from build123d import *

# Parameters (mm, degrees)
F0_R     = 3
F1_DEPTH = 0.8
F3_DEPTH = 2


with BuildPart() as f1:
    # F0 (on Top) → F1 (new body)
    with BuildSketch(Plane.XY):
        with BuildLine():
            Line((-2, 10.345446), (0, 10.345446))
            Line((0, 10.345446), (2, 10.345446))
            Line((2, 10.345446), (5.554248, 10.345446))
            Line((5.554248, 10.345446), (16, 10.345446))
            Line((16, 10.345446), (26.5, -2.654554))
            Line((26.5, -2.654554), (28.31125, -0.122547))
            Line((28.31125, -0.122547), (18.033634, 12.60212))
            ThreePointArc((18.033634, 12.60212), (17.339915, 13.150071), (16.477752, 13.345446))
            Line((16.477752, 13.345446), (0, 13.345446))
            Line((0, 13.345446), (-16.477752, 13.345446))
            ThreePointArc((-16.477752, 13.345446), (-17.339915, 13.150071), (-18.033634, 12.60212))
            Line((-18.033634, 12.60212), (-28.31125, -0.122547))
            Line((-28.31125, -0.122547), (-26.5, -2.654554))
            Line((-26.5, -2.654554), (-16, 10.345446))
            Line((-16, 10.345446), (-5.554248, 10.345446))
            Line((-5.554248, 10.345446), (-2, 10.345446))
        make_face()
        with Locations((0, 1.345446)):
            Circle(F0_R)
    extrude(amount=F1_DEPTH)

    # F2 (on face) → F3 (join)
    with BuildSketch(Plane(origin=(0, 0, 0), x_dir=(1, 0, 0), z_dir=(0, 0, -1))):
        with BuildLine():
            Line((-26.5, 2.654554), (-28.31125, 0.122547))
            Line((-28.31125, 0.122547), (-18.033634, -12.60212))
            ThreePointArc((-18.033634, -12.60212), (-17.339915, -13.150071), (-16.477752, -13.345446))
            Line((-16.477752, -13.345446), (16.477752, -13.345446))
            ThreePointArc((16.477752, -13.345446), (17.339915, -13.150071), (18.033634, -12.60212))
            Line((18.033634, -12.60212), (28.31125, 0.122547))
            Line((28.31125, 0.122547), (26.5, 2.654554))
            Line((26.5, 2.654554), (-26.5, 2.654554))
        make_face()
    extrude(amount=F3_DEPTH)


solid = f1.part
Source: CAD feature listing. Evaluate the final solid. Frame: model axes, mm. A direction names the side the tool comes from. Give positions to 0.01 mm unless a question says otherwise; leave off trailing zeros. Order: outer loops, then holes, each group sorted by start corner. A loop starts at its lowest first (then second) coordinate and runs counter-clockwise, first axis right, second up. Notation, with made-up numbers: (64.25, 81.25) -> (97.25, 81.25) arc R21 ccw to (97.25, 96.25) -> close; hole circle Ø3 at (39, 14.25). An arc over 180 degrees is marked (long way). Use a Markdown table: item, result.
1) Section query C-C, the plane x = -21.5. Return the cut outline in (y, z), then the cut area to 3 significant figures.
Answer list:
| item | result |
|---|---|
| outline | (-2.65, -2) -> (8.31, -2) -> (8.31, 0.8) -> (3.54, 0.8) -> (3.54, 0) -> (-2.65, 0) -> close |
| area | 25.7 mm² |
2) Mould query, pull axis X, two halves, no side actions, for faces 3 (the cylindrical face through (-0.65, -1.583, 0.394)), 4 (the flat face through (-23.244, 6.151, -0.58)), 5 (the flat face through (0, -2.655, -1)). Classes: +X half, -X half, draft (parallel to the pull), parting line (faces both ways), or undercut.
Answer list:
| item | result |
|---|---|
| face 3 | undercut |
| face 4 | -X half |
| face 5 | draft |
3) Section query A-A, the plane x = 0. Return the cut outline in (y, z).
Answer list:
| item | result |
|---|---|
| outline | (-2.65, -2) -> (13.35, -2) -> (13.35, 0.8) -> (10.35, 0.8) -> (10.35, 0) -> (4.35, 0) -> (4.35, 0.8) -> (-1.65, 0.8) -> (-1.65, 0) -> (-2.65, 0) -> close |
4) Section query B-B, the plane y = 7. Return the cut outline in (x, z), then the cut area to 3 significant figures.
Answer list:
| item | result |
|---|---|
| outline | (-22.56, -2) -> (22.56, -2) -> (22.56, 0.8) -> (18.7, 0.8) -> (18.7, 0) -> (-18.7, 0) -> (-18.7, 0.8) -> (-22.56, 0.8) -> close |
| area | 96.4 mm² |
5) Contact query for flat-ended pins moving along their axis: P1, Ø1, axis at y = 1.5, z = 0, coming from the +X side; P2, Ø1, axis at x = -3.5, y = 5.5, coming from the +Z side. Output: stop coordinate, or through.
Answer list:
| item | result |
|---|---|
| P1 | x = 27.4 |
| P2 | z = 0 |
6) Reachability of faces 1 (the flat face through (0, 5, -2)), 2 (the flat face through (21.176, 3.936, 0.394)) from +Z, -Z, +X, -X, +Y, -Y: full face, straight path, thin tool, end or side. Return the list, or none.
Answer list:
| item | result |
|---|---|
| face 1 | -Z, +X, -X, +Y, -Y |
| face 2 | +Z, -Y |
7) Ray query, line 1 along X through (y, z) = (3.25, 0.15); line 2 along Y through (x, z) = (13.5, 0.6); line 3 along Z through (x, y) = (2.5, 6.75). Return the intervals inside material, ascending. Write a range as [from, to].
Answer list:
| item | result |
|---|---|
| line 1 | [-25.59, -21.73], [-2.32, 2.32], [21.73, 25.59] |
| line 2 | [10.35, 13.35] |
| line 3 | [-2, 0] |
8) Section query D-D, the plane x = 21. Return the cut outline in (y, z).
Answer list:
| item | result |
|---|---|
| outline | (-2.65, -2) -> (8.93, -2) -> (8.93, 0.8) -> (4.15, 0.8) -> (4.15, 0) -> (-2.65, 0) -> close |
